Design review of the part built by this model. Coordinates are the model's own, in mm. Face numbers are marked on the shaded views. A direction names the side the tool comes from. Give positions to 0.01 mm unless a question says otherwise; leave off trailing zeros. Order: outer loops, then holes, each group sorted by start corner. A loop starts at its lowest first (then second) coordinate and runs counter-clockwise, first axis right, second up. Notation, with made-up numbers: (37.5, 14) -> (86.5, 14) arc R17 ccw to (86.5, 41) -> close; hole circle Ø3 at (20, 28.25). An arc over 180 degrees is marked (long way). Return JSON: item names as keys, results as strings.
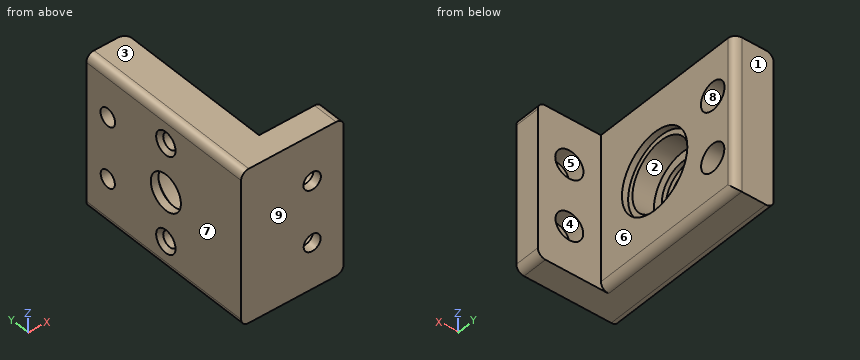
```python
from build123d import *

# Parameters (mm, degrees)
SKETCH1_W               = 20
SKETCH1_H               = 30
BOSS_EXTRUDE1_DEPTH     = 5
SKETCH2_W               = 7.7
SKETCH2_H               = 30
BOSS_EXTRUDE2_DEPTH     = 25
CUT_EXTRUDE1_DEPTH      = 36.725201189
CUT_EXTRUDE1_DEPTH_BACK = 36.725201189
SKETCH3_R               = 3.5
SKETCH4_R               = 7.6
CUT_EXTRUDE2_DEPTH      = 1.2
SKETCH5_R               = 6.6
CUT_EXTRUDE3_DEPTH      = 4.2
SKETCH6_R               = 4.75
CUT_EXTRUDE4_DEPTH      = 0.8
CUT_EXTRUDE5_DEPTH      = 31.822070015
CUT_EXTRUDE5_DEPTH_BACK = 31.822070015
SKETCH7_R               = 1.65
SKETCH7_R_2             = 1.7
SKETCH8_R               = 2.7
CUT_EXTRUDE6_DEPTH      = 3.2
SKETCH9_R               = 2.75
CUT_EXTRUDE7_DEPTH      = 3.3
SKETCH10_W              = 7.7
SKETCH10_H              = 30
BOSS_EXTRUDE3_DEPTH     = 6
CUT_EXTRUDE8_DEPTH      = 41.893642538
CUT_EXTRUDE8_DEPTH_BACK = 41.893642538
SKETCH11_R              = 1.7
SKETCH11_R_2            = 1.65
SKETCH12_R              = 2.7
CUT_EXTRUDE9_DEPTH      = 3.2
SKETCH13_R              = 2.75
CUT_EXTRUDE10_DEPTH     = 3.3
SKETCH14_R              = 1.5
CUT_EXTRUDE11_DEPTH     = 4.5
CHAMFER1_SIZE           = 0.75
FILLET1_R               = 1.5


with BuildPart() as part:
    # Sketch1 → Boss-Extrude1 (new body)
    with BuildSketch(Plane(origin=(0, 0, 0), x_dir=(1, 0, 0), z_dir=(0, 1, 0))):
        Rectangle(SKETCH1_W, SKETCH1_H)
    extrude(amount=BOSS_EXTRUDE1_DEPTH)

    # Sketch2 → Boss-Extrude2 (add)
    with BuildSketch(Plane(origin=(0, 5, 0), x_dir=(1, 0, 0), z_dir=(0, 1, 0))):
        with Locations((-6.15, 0)):
            Rectangle(SKETCH2_W, SKETCH2_H)
    extrude(amount=BOSS_EXTRUDE2_DEPTH)

    # Sketch3 → Cut-Extrude1 (cut, two sides: drawn at the far end of the back side and taken through both)
    with BuildSketch(Plane(origin=(-2.3, 0, 0), x_dir=(0, 0, -1), z_dir=(1, 0, 0)).offset(-CUT_EXTRUDE1_DEPTH_BACK)):
        with Locations((0, 17.5)):
            Circle(SKETCH3_R)
    extrude(amount=CUT_EXTRUDE1_DEPTH + CUT_EXTRUDE1_DEPTH_BACK, mode=Mode.SUBTRACT)

    # Sketch4 → Cut-Extrude2 (cut)
    with BuildSketch(Plane(origin=(-2.3, 0, 0), x_dir=(0, 0, -1), z_dir=(1, 0, 0))):
        with Locations((0, 17.5)):
            Circle(SKETCH4_R)
    extrude(amount=-CUT_EXTRUDE2_DEPTH, mode=Mode.SUBTRACT)

    # Sketch5 → Cut-Extrude3 (cut)
    with BuildSketch(Plane(origin=(-3.5, 0, 0), x_dir=(0, 0, -1), z_dir=(1, 0, 0))):
        with Locations((0, 17.5)):
            Circle(SKETCH5_R)
    extrude(amount=-CUT_EXTRUDE3_DEPTH, mode=Mode.SUBTRACT)

    # Sketch6 → Cut-Extrude4 (cut)
    with BuildSketch(Plane(origin=(-7.7, 0, 0), x_dir=(0, 0, -1), z_dir=(1, 0, 0))):
        with Locations((0, 17.5)):
            Circle(SKETCH6_R)
    extrude(amount=-CUT_EXTRUDE4_DEPTH, mode=Mode.SUBTRACT)

    # Sketch7 → Cut-Extrude5 (cut, two sides: drawn at the far end of the back side and taken through both)
    with BuildSketch(Plane(origin=(0, 5, 0), x_dir=(1, 0, 0), z_dir=(0, 1, 0)).offset(-CUT_EXTRUDE5_DEPTH_BACK)):
        with Locations(Location((3.85, 6, 0), (0, 0, 270))):
            Circle(SKETCH7_R)
        with Locations(Location((3.85, -6, 0), (0, 0, 270))):
            Circle(SKETCH7_R_2)
    extrude(amount=CUT_EXTRUDE5_DEPTH + CUT_EXTRUDE5_DEPTH_BACK, mode=Mode.SUBTRACT)

    # Sketch8 → Cut-Extrude6 (cut)
    with BuildSketch(Plane(origin=(0, 5, 0), x_dir=(1, 0, 0), z_dir=(0, 1, 0))):
        with Locations(Location((3.85, 6, 0), (0, 0, 270))):
            Circle(SKETCH8_R)
    extrude(amount=-CUT_EXTRUDE6_DEPTH, mode=Mode.SUBTRACT)

    # Sketch9 → Cut-Extrude7 (cut)
    with BuildSketch(Plane(origin=(0, 5, 0), x_dir=(1, 0, 0), z_dir=(0, 1, 0))):
        with Locations(Location((3.85, -6, 0), (0, 0, 270))):
            Circle(SKETCH9_R)
    extrude(amount=-CUT_EXTRUDE7_DEPTH, mode=Mode.SUBTRACT)

    # Sketch10 → Boss-Extrude3 (add)
    with BuildSketch(Plane(origin=(0, 30, 0), x_dir=(1, 0, 0), z_dir=(0, 1, 0))):
        with Locations((-6.15, 0)):
            Rectangle(SKETCH10_W, SKETCH10_H)
    extrude(amount=BOSS_EXTRUDE3_DEPTH)

    # Sketch11 → Cut-Extrude8 (cut, two sides: drawn at the far end of the back side and taken through both)
    with BuildSketch(Plane(origin=(-2.3, 0, 0), x_dir=(0, 0, -1), z_dir=(1, 0, 0)).offset(-CUT_EXTRUDE8_DEPTH_BACK)):
        with Locations((-6, 31)):
            Circle(SKETCH11_R)
        with Locations((6, 31)):
            Circle(SKETCH11_R_2)
    extrude(amount=CUT_EXTRUDE8_DEPTH + CUT_EXTRUDE8_DEPTH_BACK, mode=Mode.SUBTRACT)

    # Sketch12 → Cut-Extrude9 (cut)
    with BuildSketch(Plane(origin=(-2.3, 0, 0), x_dir=(0, 0, -1), z_dir=(1, 0, 0))):
        with Locations((6, 31)):
            Circle(SKETCH12_R)
    extrude(amount=-CUT_EXTRUDE9_DEPTH, mode=Mode.SUBTRACT)

    # Sketch13 → Cut-Extrude10 (cut)
    with BuildSketch(Plane(origin=(-2.3, 0, 0), x_dir=(0, 0, -1), z_dir=(1, 0, 0))):
        with Locations((-6, 31)):
            Circle(SKETCH13_R)
    extrude(amount=-CUT_EXTRUDE10_DEPTH, mode=Mode.SUBTRACT)

    # Sketch14 → Cut-Extrude11 (cut)
    with BuildSketch(Plane.ZY.offset(10)):
        with Locations((-9.525, 17.5)):
            Circle(SKETCH14_R)
        with Locations((9.525, 17.5)):
            Circle(SKETCH14_R)
    extrude(amount=-CUT_EXTRUDE11_DEPTH, mode=Mode.SUBTRACT)

    # Chamfer1
    chamfer1_edges = [part.edges().sort_by_distance(p)[0] for p in [
        (-10, 17.5, -11.025),
        (-10, 17.5, 8.025),
    ]]
    chamfer(chamfer1_edges, length=CHAMFER1_SIZE)

    # Fillet1
    fillet1_edges = [part.edges().sort_by_distance(p)[0] for p in [
        (-2.3, 20.5, -15),
        (10, 2.5, 15),
        (-10, 18, 15),
        (-10, 18, -15),
        (-2.3, 36, 0),
        (10, 2.5, -15),
    ]]
    fillet(fillet1_edges, radius=FILLET1_R)


solid = part.part
```
Item 1: Add section C-C (y = 26). Give the boundary of the cut face in (x, z).
Result set:
{"outline": "(-10, -13.5) arc R1.5 ccw to (-8.5, -15) -> (-3.8, -15) arc R1.5 ccw to (-2.3, -13.5) -> (-2.3, 15) -> (-8.5, 15) arc R1.5 ccw to (-10, 13.5) -> close"}
Item 2: Add section B-B (z = 0). Give the boundary of the cut face in (x, y), plus the area to 3 significant figures.
Result set:
{"outline": "(-10, 0) -> (10, 0) -> (10, 5) -> (-2.3, 5) -> (-2.3, 9.9) -> (-3.5, 9.9) -> (-3.5, 10.9) -> (-7.7, 10.9) -> (-7.7, 12.75) -> (-8.5, 12.75) -> (-8.5, 14) -> (-10, 14) -> close; (-10, 21) -> (-8.5, 21) -> (-8.5, 22.25) -> (-7.7, 22.25) -> (-7.7, 24.1) -> (-3.5, 24.1) -> (-3.5, 25.1) -> (-2.3, 25.1) -> (-2.3, 34.5) arc R1.5 ccw to (-3.8, 36) -> (-10, 36) -> close", "area": "246 mm^2"}
Item 3: For pin 1 (5 mm diameter, centred on y = 17.5, z = 9.525, fed in from +X); pin 2 (1.5 mm diameter, centred on x = -1, y = 12.5, fed in from -Z); pin 3 (8 mm diameter, centred on x = 2, z = -5, fed in from -Y); pin 4 (4 mm diameter, centred on x = 0, z = 0, fed in from +Y), all flat-tipped, find the tip position at first contact; note any pin that passes through.
Result set:
{"pin 1": "stops at x = -2.3", "pin 2": "passes through", "pin 3": "stops at y = 0", "pin 4": "stops at y = 5"}
Item 4: Add section A-A (x = 3.85). Give the boundary of the cut face in (y, z), plus the area to 3 significant figures.
Result set:
{"outline": "(0, -15) -> (5, -15) -> (5, -8.7) -> (1.8, -8.7) -> (1.8, -7.65) -> (0, -7.65) -> close; (0, -4.35) -> (1.8, -4.35) -> (1.8, -3.3) -> (5, -3.3) -> (5, 3.25) -> (1.7, 3.25) -> (1.7, 4.3) -> (0, 4.3) -> close; (0, 7.7) -> (1.7, 7.7) -> (1.7, 8.75) -> (5, 8.75) -> (5, 15) -> (0, 15) -> close", "area": "103 mm^2"}
Item 5: Wall thickness on L1, parallel to Z at x = 3.85, y = 1.25; L2, parallel to X at y = 1.3, z = -6; L3, parallel to Y at x = -7.5, z = -5.5: over which ranges is each line inside the solid? List them lowest first. Write a range as [from, to].
Result set:
{"L1": "z = [-15, -7.65], [-4.35, 4.3], [7.7, 15]", "L2": "x = [-10, 2.2], [5.5, 10]", "L3": "y = [0, 13.85], [21.15, 29.43], [32.57, 36]"}
Item 6: Machinability: for the marked faces 5, 6, 7, 8 and 9, which of the approach directions +Z, -Z, +X, -X, +Y, -Y give a long, thin tool a straight path to every point of the face, cutting with its end or side? Answer none if there is none.
Result set:
{"face 5": "+Y", "face 6": "+Z, -Z, +X, +Y", "face 7": "+Z, -Z, -X, +Y, -Y", "face 8": "+X", "face 9": "+Z, -Z, +X, -X, -Y"}
Item 7: Mouldability with a two-part tool opening along Z and no side actions: class the marked faces 1, 2, 3 and 4 as released by +Z, released by -Z, zero draft, split by the parting line, or undercut.
Result set:
{"face 1": "zero draft", "face 2": "undercut", "face 3": "released by +Z", "face 4": "undercut"}
Item 8: Add section D-D (x = -4.75). Give the boundary of the cut face in (y, z).
Result set:
{"outline": "(0, -15) -> (36, -15) -> (36, 15) -> (0, 15) -> close; hole circle Ø13.2 at (17.5, 0); hole circle Ø5.5 at (31, 6); hole circle Ø5.4 at (31, -6)"}
